The drawing under review shows one solid part. Ordinate dimensions are in mm from its lowest x, y, z. Coordinates: 2 decimals unless noted, no trailing zeros. Order: outer loops, then holes, each group sorted by start corner. A loop starts at its lowest first (then second) coordinate and runs counter-clockwise, first axis right, second up. Notation, with made-up numbers: M 82,-10 L 104,-10 A23 ccw 104,8 Z; hole C 25.25,-31.5 d7. An arc over 180 degrees is marked long. Answer as a JSON object with one key per item and string values.
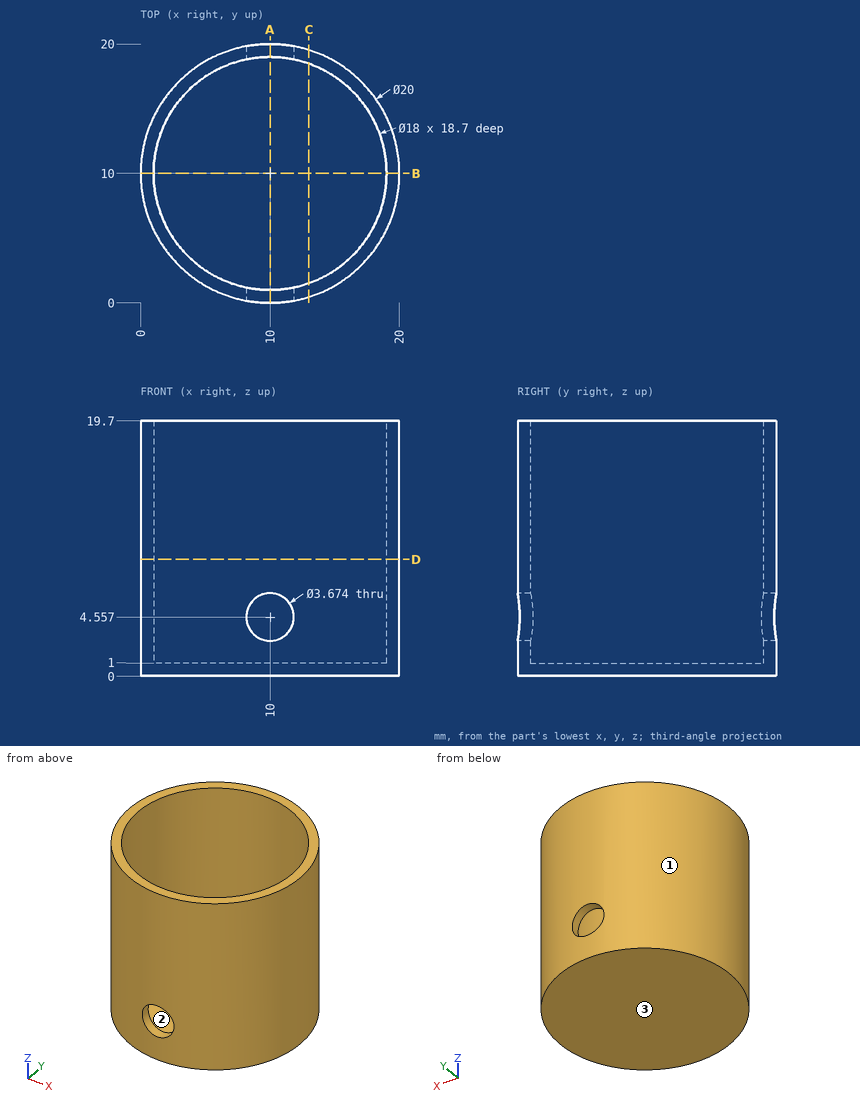
1) Add section D-D (z = 9). State the section outline as (x, y) points.
Taken from the geometry:
{"outline": "C 10,10 d20; hole C 10,10 d18"}
2) Mouldability with a two-part tool opening along X and no side actions: class the marked faces 1, 2 and 3 as released by +X, released by -X, zero draft, split by the parting line, or undercut.
Taken from the geometry:
{"face 1": "split by the parting line", "face 2": "undercut", "face 3": "zero draft"}
3) To check wall thickness, follow L1, parallel to Y at x = 10, z = 11.25; L2, parallel to Z at x = 10, y = 19.4; L3, parallel to Z at x = 14, y = 5. State the ranges of each line that lie inside material, in increasing order.
Taken from the geometry:
{"L1": "y = 0 to 1, 19 to 20", "L2": "z = 0 to 2.72, 6.39 to 19.7", "L3": "z = 0 to 1"}
4) Add section C-C (x = 13). State the section outline as (y, z) points, and give its area (3 significant figures).
Taken from the geometry:
{"outline": "M 0.46,0 L 19.54,0 L 19.54,19.7 L 18.49,19.7 L 18.49,1 L 1.51,1 L 1.51,19.7 L 0.46,19.7 Z", "area": "58.5 mm2"}
5) Insertion check: pin 1 Ø5 at (y, z) = (4, 9) entering from +X; pin 2 Ø1.5 at (x, y) = (3.5, 11.5) entering from +Z; pin 3 Ø1 at (y, z) = (16, 16) entering from -X. Each pin has a flat end and moves straight along its axis. Give the tip position at first contact, or say it passes through.
Taken from the geometry:
{"pin 1": "stops at x = 19.37", "pin 2": "stops at z = 1", "pin 3": "stops at x = 1.65"}
6) Add section B-B (y = 10). State the section outline as (x, z) points.
Taken from the geometry:
{"outline": "M 0,0 L 20,0 L 20,19.7 L 19,19.7 L 19,1 L 1,1 L 1,19.7 L 0,19.7 Z"}
7) Add section A-A (x = 10). State the section outline as (y, z) points.
Taken from the geometry:
{"outline": "M 0,0 L 20,0 L 20,2.72 L 19,2.72 L 19,1 L 1,1 L 1,2.72 L 0,2.72 Z; M 0,6.39 L 1,6.39 L 1,19.7 L 0,19.7 Z; M 19,6.39 L 20,6.39 L 20,19.7 L 19,19.7 Z"}
